from build123d import *

# Parameters (mm, degrees)
F1_DEPTH = 12.192
F3_W     = 260.35
F3_H     = 21.6032387971
F4_DEPTH = 12.192
F5_W     = 260.35
F5_H     = 21.59
F6_DEPTH = 12.192
F7_R     = 12.7


with BuildPart() as f1:
    # F0 (on Front) → F1 (new body)
    with BuildSketch(Plane.XZ):
        Polygon((115.4489097687, 44.9104134451), (-8.7127741426, 44.9104134451), (-8.7127741426, 12.2448502547), (115.4489097687, 12.2448502547), (115.4489097687, 28.5776318499), align=None)
        with BuildLine():
            add(Edge.make_bspline(
                [(-201.3751125628, 28.5776318499), (-203.6036875056, 28.2155507261), (-213.5160050083, 24.8398299044), (-212.7768922816, 16.2961456434), (-212.3699930733, 11.8833564186)],
                knots=[0.1713367735, 0.1713367735, 0.1713367735, 0.1713367735, 0.5720981619, 1, 1, 1, 1], degree=3))
            Line((-201.3751125628, 28.5776318499), (-249.5887362649, 28.5776318499))
            add(Edge.make_bspline(
                [(-249.5887362649, 28.5776318499), (-245.3983662499, 26.3811930315), (-236.7722226078, 21.8596837899), (-234.7906912251, 11.49704289), (-233.7717394185, 6.1683199847)],
                knots=[0, 0, 0, 0, 0.4857755898, 1, 1, 1, 1], degree=3))
            Line((-233.7717394185, 6.1683199847), (-224.7518429065, -40.4246754655))
            Line((-224.7518429065, -40.4246754655), (-212.3699930733, -40.4246754655))
            Line((-212.3699930733, -40.4246754655), (-212.3699930733, 11.8833564186))
        make_face()
        with BuildLine():
            add(Edge.make_bspline(
                [(232.1631879797, 28.5776318499), (227.9728179646, 26.3811930315), (219.3466743226, 21.8596837899), (217.3651429399, 11.49704289), (216.3461911332, 6.1683199847)],
                knots=[0, 0, 0, 0, 0.4857755898, 1, 1, 1, 1], degree=3))
            Line((232.1631879797, 28.5776318499), (183.9495642776, 28.5776318499))
            add(Edge.make_bspline(
                [(183.9495642776, 28.5776318499), (186.1781392203, 28.2155507261), (196.0904567231, 24.8398299044), (195.3513439963, 16.2961456434), (194.944444788, 11.8833564186)],
                knots=[0.1713367735, 0.1713367735, 0.1713367735, 0.1713367735, 0.5720981619, 1, 1, 1, 1], degree=3))
            Line((194.944444788, 11.8833564186), (194.944444788, -40.4246754655))
            Line((194.944444788, -40.4246754655), (207.3262946213, -40.4246754655))
            Line((207.3262946213, -40.4246754655), (216.3461911332, 6.1683199847))
        make_face()
        with BuildLine():
            Line((-132.874458054, 12.2448502547), (-132.874458054, 28.5776318499))
            Line((-132.874458054, 28.5776318499), (-160.3592138582, 28.5776318499))
            Line((-160.3592138582, 28.5776318499), (-160.3592138582, -40.1182342476))
            Line((-160.3592138582, -40.1182342476), (-143.3239786863, -40.1182342476))
            Line((-143.3239786863, -40.1182342476), (-139.2062762381, 9.481767078))
            ThreePointArc((-139.2062762381, 9.481767078), (-136.3286783046, 11.5239959202), (-132.874458054, 12.2448502547))
        make_face()
        with BuildLine():
            Line((115.4489097687, 28.5776318499), (115.4489097687, 12.2448502547))
            ThreePointArc((115.4489097687, 12.2448502547), (118.9031300193, 11.5239959202), (121.7807279529, 9.481767078))
            Line((121.7807279529, 9.481767078), (125.898430401, -40.1182342476))
            Line((125.898430401, -40.1182342476), (142.933665573, -40.1182342476))
            Line((142.933665573, -40.1182342476), (142.933665573, 28.5776318499))
            Line((142.933665573, 28.5776318499), (115.4489097687, 28.5776318499))
        make_face()
        with BuildLine():
            Line((115.4489097687, 50.180870647), (115.4489097687, 44.9104134451))
            Line((115.4489097687, 44.9104134451), (115.4489097687, 28.5776318499))
            Line((115.4489097687, 28.5776318499), (142.933665573, 28.5776318499))
            Line((142.933665573, 28.5776318499), (182.0295738914, 28.5776318499))
            add(Edge.make_bspline(
                [(182.0295738914, 28.5776318499), (182.5128861487, 28.6550095059), (182.9967857635, 28.7324317216), (183.9495642776, 28.5776318499)],
                knots=[0, 0, 0, 0, 0.1713367735, 0.1713367735, 0.1713367735, 0.1713367735], degree=3))
            Line((183.9495642776, 28.5776318499), (232.1631879797, 28.5776318499))
            Line((232.1631879797, 28.5776318499), (252.4502187865, 28.5776318499))
            Line((252.4502187865, 28.5776318499), (252.4502187865, 50.180870647))
            Line((252.4502187865, 50.180870647), (115.4489097687, 50.180870647))
        make_face()
        Polygon((-8.7127741426, 44.9104134451), (-132.874458054, 44.9104134451), (-132.874458054, 28.5776318499), (-132.874458054, 12.2448502547), (-8.7127741426, 12.2448502547), align=None)
        with BuildLine():
            Line((-132.874458054, 28.5776318499), (-132.874458054, 44.9104134451))
            Line((-132.874458054, 44.9104134451), (-132.874458054, 50.180870647))
            Line((-132.874458054, 50.180870647), (-269.8757670717, 50.180870647))
            Line((-269.8757670717, 50.180870647), (-269.8757670717, 28.5776318499))
            Line((-269.8757670717, 28.5776318499), (-249.5887362649, 28.5776318499))
            Line((-249.5887362649, 28.5776318499), (-201.3751125628, 28.5776318499))
            add(Edge.make_bspline(
                [(-199.4551221767, 28.5776318499), (-199.9384344339, 28.6550095059), (-200.4223340487, 28.7324317216), (-201.3751125628, 28.5776318499)],
                knots=[0, 0, 0, 0, 0.1713367735, 0.1713367735, 0.1713367735, 0.1713367735], degree=3))
            Line((-199.4551221767, 28.5776318499), (-160.3592138582, 28.5776318499))
            Line((-160.3592138582, 28.5776318499), (-132.874458054, 28.5776318499))
        make_face()
        with BuildLine():
            add(Edge.make_bspline(
                [(182.0295738914, 28.5776318499), (182.5128861487, 28.6550095059), (182.9967857635, 28.7324317216), (183.9495642776, 28.5776318499)],
                knots=[0, 0, 0, 0, 0.1713367735, 0.1713367735, 0.1713367735, 0.1713367735], degree=3))
            Line((182.0295738914, 28.5776318499), (183.9495642776, 28.5776318499))
        make_face()
        with BuildLine():
            Line((-201.3751125628, 28.5776318499), (-199.4551221767, 28.5776318499))
            add(Edge.make_bspline(
                [(-199.4551221767, 28.5776318499), (-199.9384344339, 28.6550095059), (-200.4223340487, 28.7324317216), (-201.3751125628, 28.5776318499)],
                knots=[0, 0, 0, 0, 0.1713367735, 0.1713367735, 0.1713367735, 0.1713367735], degree=3))
        make_face()
    extrude(amount=F1_DEPTH)


with BuildPart() as f2_1:
    # F2: copy of F1
    add(f1.part.moved(Location((0, -248.158, 0))))


with BuildPart() as f1_1:
    add(f1.part)

    add(f2_1.part)  # F4 merges F2_1
    # F3 (on face) → F4 (join)
    with BuildSketch(Plane.YZ.offset(252.4502187865)):
        with Locations((-130.175, 39.3792512485)):
            Rectangle(F3_W, F3_H)
    extrude(amount=F4_DEPTH)

    # F5 (on face) → F6 (join)
    with BuildSketch(Plane(origin=(-269.8757670717, 0, 0), x_dir=(0, -1, 0), z_dir=(-1, 0, 0))):
        with Locations((130.175, 39.385870647)):
            Rectangle(F5_W, F5_H)
    extrude(amount=F6_DEPTH)

    # F7
    f7_edges = [f1_1.edges().sort_by_distance(p)[0] for p in [
        (264.642219, -260.35, 39.379251),
        (264.642219, 0, 39.379251),
        (-282.067767, 0, 39.385871),
        (-282.067767, -260.35, 39.385871),
        (252.450219, -12.192, 39.379251),
        (252.450219, -248.158, 39.379251),
        (-269.875767, -248.158, 39.385871),
        (-269.875767, -12.192, 39.385871),
    ]]
    fillet(f7_edges, radius=F7_R)


solid = f1_1.part
Model file for the job. Use its own axes, mm. A direction names the side the tool comes from. Round coordinates to 2 decimals unless told otherwise and drop trailing zeros. Loops run counter-clockwise (first coordinate to the right, second up) from the corner with the lowest first, then second, coordinate; pieces in that order, holes last. Notation, with made-up numbers: (49.5, 83) - (102.5, 83) arc R20 cw to (102.5, 110) - close; hole circle Ø8 at (-1.5, -5). An arc over 180 degrees is marked (long way). Write each question's results on one line, items separated by ' | '.
(1) Saw through at B-B, the plane y = -208. List the corners of the cut face in (x, z).
Answer below:
outline: (-282.07, 28.59) - (-269.88, 28.59) - (-269.88, 50.18) - (-282.07, 50.18) - close; (252.45, 28.58) - (264.64, 28.58) - (264.64, 50.18) - (252.45, 50.18) - close
(2) Mould opens along Y. For faces 4 (the cylindrical face through (248.83, -244.34, 39.53)), 5 (the flat face through (-10, -6, 12.245)) say: released by +Y, released by -Y, zero draft, split by the parting line, or undercut.
Answer below:
face 4: undercut | face 5: zero draft
(3) Saw through at C-C, the plane z = -21. Count the separate pieces of the cut face and the enclosed holes in it, then the cut area to 3 significant figures.
Answer below:
separate pieces: 8 | enclosed holes: 0 | area: 1,700 mm^2
(4) Pin check, flat tips, straight feed: pin 1 (13.5 mm diameter, centred on x = -8, y = -254.5, fed in from +Z); pin 2 (10 mm diameter, centred on x = 170, y = -6.5, fed in from -Z); pin 3 (6 mm diameter, centred on y = -256, z = -16, fed in from -X). Stop position of each tip, or through.
Answer below:
pin 1: stops at z = 44.91 | pin 2: stops at z = 28.58 | pin 3: stops at x = -230.06
(5) Saw through at A-A, the plane x = 159.5. List the corners of the cut face in (y, z), then the cut area to 3 significant figures.
Answer below:
outline: (-260.35, 28.58) - (-248.16, 28.58) - (-248.16, 50.18) - (-260.35, 50.18) - close; (-12.19, 28.58) - (0, 28.58) - (0, 50.18) - (-12.19, 50.18) - close | area: 527 mm^2
(6) 3-axis set-ups, long thin cutter, end or side, ignore diameter. For faces 1 (the flat face through (-10, -254, 12.245)), 2 (the flat face through (-7, -6, 44.91)), 3 (the flat face through (38, -248.158, 26)): which of +Z, -Z, +X, -X, +Y, -Y reach the whole face in a straight line?
Answer below:
face 1: -Z, +Y, -Y | face 2: +Z, +Y, -Y | face 3: +Z, -Z
(7) Wall check: L1, parallel to X at y = -127, z = 44.5; L2, parallel to Y at x = -146, z = 19. Give the ranges that are in metal, low to high.
Answer below:
L1: x = -282.07 to -269.88, 252.45 to 264.64 | L2: y = -260.35 to -248.16, -12.19 to 0
